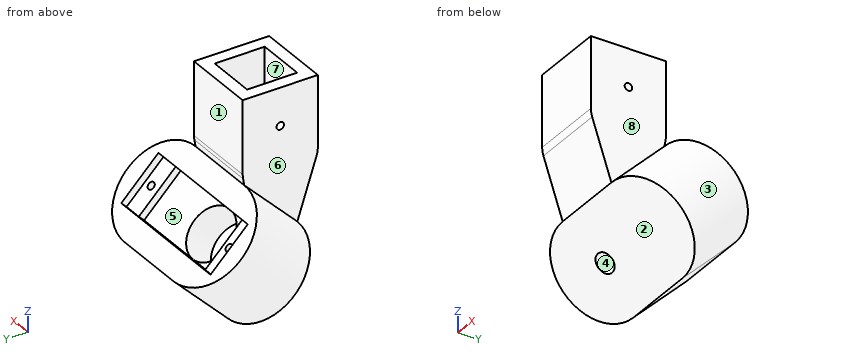
from build123d import *

# Parameters (mm, degrees)
SKETCH1_W           = 30
SKETCH1_H           = 30
BOSS_EXTRUDE1_DEPTH = 30
BOSS_EXTRUDE3_DEPTH = 30
SKETCH19_W          = 55
SKETCH19_H          = 21
CUT_EXTRUDE2_DEPTH  = 3
SKETCH20_R          = 1.5
CUT_EXTRUDE3_DEPTH  = 10
SKETCH21_R          = 10.5
CUT_EXTRUDE4_DEPTH  = 30
SKETCH22_W          = 40.9
SKETCH22_H          = 21
CUT_EXTRUDE7_DEPTH  = 3
FILLET2_R           = 10
FILLET3_R           = 10
SKETCH23_R          = 1.5
CUT_EXTRUDE8_DEPTH  = 30
SKETCH24_W          = 23.993806076
SKETCH24_H          = 21.426788773
SKETCH24_R          = 4
BOSS_EXTRUDE4_DEPTH = 10
SKETCH25_W          = 20
SKETCH25_H          = 20
CUT_EXTRUDE10_DEPTH = 30


with BuildPart() as part:
    # Sketch1 → Boss-Extrude1 (new body)
    with BuildSketch(Plane.XY):
        Rectangle(SKETCH1_W, SKETCH1_H)
        Polygon((-3.181061689, 4.218151635), (-0.042296032, 4.218151635), (3.181061689, 4.218151635), (5.633333333, 6.670423279), (5.633333333, 8.284397195), (2.733333333, 8.284397195), (2.733333333, 10), (10, 10), (10, 2.733333333), (8.80386145, 2.733333333), (8.80386145, 5.633333333), (6.670423279, 5.633333333), (4.218151635, 3.181061689), (4.218151635, 0.042296032), (4.218151635, -3.181061689), (6.670423279, -5.633333333), (8.284397195, -5.633333333), (8.284397195, -2.733333333), (10, -2.733333333), (10, -10), (2.733333333, -10), (2.733333333, -8.80386145), (5.633333333, -8.80386145), (5.633333333, -6.670423279), (3.181061689, -4.218151635), (0.042296032, -4.218151635), (-3.181061689, -4.218151635), (-5.633333333, -6.670423279), (-5.633333333, -8.284397195), (-2.733333333, -8.284397195), (-2.733333333, -10), (-10, -10), (-10, -2.733333333), (-8.80386145, -2.733333333), (-8.80386145, -5.633333333), (-6.670423279, -5.633333333), (-4.218151635, -3.181061689), (-4.218151635, -0.042296032), (-4.218151635, 3.181061689), (-6.670423279, 5.633333333), (-8.284397195, 5.633333333), (-8.284397195, 2.733333333), (-10, 2.733333333), (-10, 10), (-2.733333333, 10), (-2.733333333, 8.80386145), (-5.633333333, 8.80386145), (-5.633333333, 6.670423279), align=None, mode=Mode.SUBTRACT)
    extrude(amount=BOSS_EXTRUDE1_DEPTH)



with BuildPart() as body_2:
    # Sketch9 → Boss-Extrude3 (new body)
    with BuildSketch(Plane(origin=(15, 17.928932188, -7.071067812), x_dir=(1, 0, 0), z_dir=(0, 0.7071067811865437, 0.7071067811865515))):
        with BuildLine():
            Line((0, -5), (-30, -5))
            ThreePointArc((-30, -5), (-50, 15), (-30, 35))
            Line((-30, 35), (0, 35))
            ThreePointArc((0, 35), (20, 15), (0, -5))
        make_face()
    extrude(amount=-BOSS_EXTRUDE3_DEPTH)


with BuildPart() as part_1:
    add(part.part)

    add(body_2.part)  # Loft5 merges body 2
    # Sketch16 → Loft5 section 0
    with BuildSketch(Plane(origin=(0, 8.964466094, -8.964466094), x_dir=(1, 0, 0), z_dir=(0, -0.7071067811865513, 0.7071067811865438))):
        with BuildLine():
            Line((-15, 7.67766953), (15, 7.67766953))
            Line((15, 7.67766953), (15, -22.32233047))
            Line((15, -22.32233047), (-15, -22.32233047))
            Line((-15, -22.32233047), (-15, 7.67766953))
        make_face()
    # Sketch17 → Loft5 section 1
    with BuildSketch(Plane(origin=(0, 0, 0), x_dir=(-1, 0, 0), z_dir=(0, 0, -1))):
        with BuildLine():
            Line((15, 15), (-15, 15))
            Line((-15, 15), (-15, -15))
            Line((-15, -15), (15, -15))
            Line((15, -15), (15, 15))
        make_face()
    loft()

    # Sketch19 → Cut-Extrude2 (cut)
    with BuildSketch(Plane(origin=(0, 5.428932188, 5.428932188), x_dir=(1, 0, 0), z_dir=(0, 0.7071067811865438, 0.7071067811865513))):
        with Locations((0, 32.67766953)):
            Rectangle(SKETCH19_W, SKETCH19_H)
    extrude(amount=-CUT_EXTRUDE2_DEPTH, mode=Mode.SUBTRACT)

    # Sketch20 → Cut-Extrude3 (cut)
    with BuildSketch(Plane(origin=(0, 3.307611845, 3.307611845), x_dir=(1, 0, 0), z_dir=(0, 0.7071067811865438, 0.7071067811865512))):
        with Locations(Location((24, 32.473176799, 0), (0, 0, 270))):
            Circle(SKETCH20_R)
        with Locations(Location((-24, 32.473176799, 0), (0, 0, 270))):
            Circle(SKETCH20_R)
    extrude(amount=-CUT_EXTRUDE3_DEPTH, mode=Mode.SUBTRACT)

    # Sketch21 → Cut-Extrude4 (cut)
    with BuildSketch(Plane(origin=(0, 3.307611845, 3.307611845), x_dir=(1, 0, 0), z_dir=(0, 0.7071067811865438, 0.7071067811865512))):
        with Locations(Location((-10, 32.67766953, 0), (0, 0, 270))):
            Circle(SKETCH21_R)
    extrude(amount=-CUT_EXTRUDE4_DEPTH, mode=Mode.SUBTRACT)

    # Sketch22 → Cut-Extrude7 (cut)
    with BuildSketch(Plane(origin=(0, 3.307611845, 3.307611845), x_dir=(1, 0, 0), z_dir=(0, 0.7071067811865438, 0.7071067811865512))):
        with Locations((-0.5, 32.67766953)):
            Rectangle(SKETCH22_W, SKETCH22_H)
    extrude(amount=-CUT_EXTRUDE7_DEPTH, mode=Mode.SUBTRACT)

    # Fillet2
    fillet2_edges = [part_1.edges().sort_by_distance(p)[0] for p in [
        (0, 15, 0),
    ]]
    fillet(fillet2_edges, radius=FILLET2_R)

    # Fillet3
    fillet3_edges = [part_1.edges().sort_by_distance(p)[0] for p in [
        (0, -15, 0),
    ]]
    fillet(fillet3_edges, radius=FILLET3_R)

    # Sketch23 → Cut-Extrude8 (cut)
    with BuildSketch(Plane(origin=(15, 0, 0), x_dir=(0, 0, -1), z_dir=(1, 0, 0))):
        with Locations(Location((-15, 0, 0), (0, 0, 90))):
            Circle(SKETCH23_R)
    extrude(amount=-CUT_EXTRUDE8_DEPTH, mode=Mode.SUBTRACT)

    # Sketch24 → Boss-Extrude4 (add)
    with BuildSketch(Plane(origin=(0, -15.784271247, -15.784271247), x_dir=(1, 0, 0), z_dir=(0, -0.7071067811865438, -0.7071067811865513))):
        with Locations((-10.45, -32.473176799)):
            Rectangle(SKETCH24_W, SKETCH24_H)
        with Locations(Location((-10.45, -32.473176799, 0), (0, 0, 270))):
            Circle(SKETCH24_R, mode=Mode.SUBTRACT)
    extrude(amount=-BOSS_EXTRUDE4_DEPTH)

    # Sketch25 → Cut-Extrude10 (cut)
    with BuildSketch(Plane.XY.offset(30)):
        Rectangle(SKETCH25_W, SKETCH25_H)
    extrude(amount=-CUT_EXTRUDE10_DEPTH, mode=Mode.SUBTRACT)


solid = part_1.part
Input: part model. Units: mm. Frame: model coordinates. Face numbers are marked on the shaded views. A direction names the side the tool comes from. Coordinates: 2 decimals unless noted, no trailing zeros. Loops run counter-clockwise (first coordinate to the right, second up) from the corner with the lowest first, then second, coordinate; pieces in that order, holes last.
Q1. Material intervals for line 1 (X direction, y = -6.5, z = 13); line 2 (Z direction, x = -5.5, y = 18), sorted ascending.
Q2. Cut plane D-D (y = 0). Give the number of separate pieces and of enclosed holes in the cut face, then the cut area to 3 significant figures.
Q3. Cut plane B-B (x = -13). Output: boundary loops of the cut face in (y, z), then the cut area to 3 significant figures.
Q4. Cut plane A-A (z = 15). Output: boundary loops of the cut face in (x, y).
Q5. Cut plane C-C (x = 2.5). Output: boundary loops of the cut face in (y, z).
Q6. Draft query along Z for the marked faces 1, 2, 3 and 4. Return one class per face: +Z half, -Z half, draft (parallel to the pull), parting line (faces both ways), or undercut.
Q7. Contact query for flat-ended pins moving along their axis: pin 1 (2 mm diameter, centred on x = -2.5, y = 15.5, fed in from -Z); pin 2 (2.5 mm diameter, centred on y = 0, z = 15, fed in from -X); pin 3 (16 mm diameter, centred on x = -0.5, z = 18.5, fed in from +Y); pin 4 (8.5 mm diameter, centred on y = 28, z = -16, fed in from +X). Output: stop coordinate, or through.
Q8. Set-up query: the marked faces 5, 6, 7 and 8. Return all of +Z, -Z, +X, -X, +Y, -Y with unobstructed straight access to the full face (end or side cutting, diameter ignored); none if empty.
Working result:
1. line 1: x = -15 to -10, 10 to 15
1. line 2: z = -49.57 to -35.43, -13.36 to -7.14
2. separate pieces: 3
2. enclosed holes: 0
2. area: 1,550 mm2
3. outline: (-15, 1.61) arc R10 ccw to (-14.49, -1.53) - (-6.82, -24.75) - (5, -36.57) - (12.07, -29.5) - (7.28, -24.7) - (17.18, -14.81) - (16.87, -14.5) - (21.11, -10.25) - (14.39, -3.54) - (14.86, -0.84) arc R10 ccw to (15, 0.85) - (15, 30) - (-15, 30) - close; (9.36, -40.93) - (21.46, -53.03) - (42.68, -31.82) - (35.96, -25.1) - (31.72, -29.34) - (31.41, -29.04) - (21.51, -38.93) - (16.43, -33.85) - close; hole circle Ø3 at (0, 15)
3. area: 2,030 mm2
4. outline: (-15, -15) - (15, -15) - (15, -1.5) - (10, -1.5) - (10, -10) - (-10, -10) - (-10, -1.5) - (-15, -1.5) - close; (-15, 1.5) - (-10, 1.5) - (-10, 10) - (10, 10) - (10, 1.5) - (15, 1.5) - (15, 15) - (-15, 15) - close
5. outline: (-15, 1.61) arc R10 ccw to (-14.49, -1.53) - (-6.82, -24.75) - (21.46, -53.03) - (42.68, -31.82) - (35.96, -25.1) - (31.72, -29.34) - (16.87, -14.5) - (21.11, -10.25) - (14.39, -3.54) - (14.86, -0.84) arc R10 ccw to (15, 0.85) - (15, 30) - (10, 30) - (10, 0) - (-10, 0) - (-10, 30) - (-15, 30) - close
6. face 1: draft
6. face 2: -Z half
6. face 3: parting line
6. face 4: undercut
7. pin 1: stops at z = -48.07
7. pin 2: passes through
7. pin 3: stops at y = 15
7. pin 4: stops at x = 35
8. face 5: none
8. face 6: +Z, -X, -Y
8. face 7: +Z
8. face 8: +Z, +X, -Y
